Read the model definition and answer for the solid it produces. Units are mm, in the model's axes. A direction names the side the tool comes from. Round coordinates to 2 decimals unless told otherwise and drop trailing zeros. Order: outer loops, then holes, each group sorted by start corner. A loop starts at its lowest first (then second) coordinate and runs counter-clockwise, first axis right, second up. Notation, with made-up numbers: (-24, 49.5) - (20, 49.5) arc R28 ccw to (20, 69.5) - close; hole circle Ø7 at (67, 17.25). An arc over 180 degrees is marked (long way). Put each result on its own line as item: value. Start each with the question number.
Q1. Which of the six approach directions +Z, -Z, +X, -X, +Y, -Y give full straight-line access (tool end or side, diameter ignored) to faces 1 (the face through (0, 0, 0)), 2 (the face through (18, -10, 17)), 3 (the face through (-14.45, 9, 47.32)), 4 (the face through (-18, 0, 33)), 5 (the face through (-0.1, 10.6, 60))?
Q2. For a pull along X with two mould halves and no side action, classify faces 6 (the face through (14.45, -9, 47.32)), 7 (the face through (-23.651, -11.715, 47.025)), 8 (the face through (5, 0, 18)), 9 (the face through (18, 0, 33)) as pulls with the +X half, pulls with the -X half, needs draft (parallel to the pull), parting line crosses it, or undercut.
Q3. Each of these flat-tipped pins is pushed along its axis until it touches: pin 1 Ø10 at (x, z) = (21.5, 52.5) entering from -Y; pin 2 Ø5 at (x, y) = (21, -6.5) entering from +Z; pin 3 Ø8 at (y, z) = (-4, 43.5) entering from -X; pin 4 Ø10.5 at (y, z) = (2.5, 53) entering from +X (3 decimals). Where does it stop, or does it pass through?
Q4. Section D-D on z = 31 is taken. Give the vertices of the cut face in (x, y), then the cut area to 3 significant figures.
Q5. Section C-C on y = -2 is taken. Give the vertices of the cut face in (x, z).
Q6. Find the intervals of material crossed by line 1 along Y through (x, z) = (-24.5, 28); line 2 along Z through (x, y) = (-14, -5.25); line 3 along X through (y, z) = (-7, 4.5), in increasing order. Write a range as from..to.
Q7. Section B-B on z = 25 is taken. Give the vertices of the cut face in (x, y).
Q8. Section A-A on x = -11 is taken. Give the vertices of the cut face in (y, z), then the cut area to 3 significant figures.
from build123d import *

# Parameters (mm, degrees)
F0_W     = 60
F0_H     = 24
F1_DEPTH = 60
F2_W     = 31
F2_H     = 20
F5_DEPTH = 25
F4_W     = 20
F4_H     = 31
F6_DEPTH = 25
F3_W     = 20
F3_H     = 31
F7_DEPTH = 25
F8_SIZE2 = 25
F8_SIZE  = 12.5
F9_R     = 3.5
F10_R    = 1


with BuildPart() as f1:
    # F0 (on Top) → F1 (new body)
    with BuildSketch(Plane.XY):
        Rectangle(F0_W, F0_H)
    extrude(amount=F1_DEPTH)

    # F2 (on face) → F5 (cut)
    with BuildSketch(Plane.XY.offset(60)):
        Rectangle(F2_W, F2_H)
    extrude(amount=-F5_DEPTH, mode=Mode.SUBTRACT)

    # F4 (on face) → F6 (cut)
    with BuildSketch(Plane(origin=(-30, 0, 0), x_dir=(0, -1, 0), z_dir=(-1, 0, 0))):
        with Locations((0, 17.5)):
            Rectangle(F4_W, F4_H)
    extrude(amount=-F6_DEPTH, mode=Mode.SUBTRACT)

    # F3 (on face) → F7 (cut)
    with BuildSketch(Plane.YZ.offset(30)):
        with Locations((0, 17.5)):
            Rectangle(F3_W, F3_H)
    extrude(amount=-F7_DEPTH, mode=Mode.SUBTRACT)

    # F8
    f8_edges = [f1.edges().sort_by_distance(p)[0] for p in [
        (30, 0, 60),
        (-30, 0, 60),
    ]]
    f8_side = f1.faces().sort_by_distance((0, -11.35378, 60))[0]
    chamfer(f8_edges, length=F8_SIZE, length2=F8_SIZE2, reference=f8_side)

    # F9
    f9_edges = [f1.edges().sort_by_distance(p)[0] for p in [
        (-17.5, 10, 33),
        (-17.5, -10, 33),
        (-17.5, -10, 2),
        (-17.5, 10, 2),
        (15.5, -10, 47.5),
        (15.5, 10, 47.5),
        (-15.5, 10, 47.5),
        (-15.5, -10, 47.5),
        (17.5, -10, 2),
        (17.5, -10, 33),
        (17.5, 10, 33),
        (17.5, 10, 2),
    ]]
    fillet(f9_edges, radius=F9_R)

    # F10
    f10_edges = [f1.edges().sort_by_distance(p)[0] for p in [
        (-30, -12, 17.5),
        (-23.75, -12, 47.5),
        (0, -12, 0),
        (0, -12, 60),
        (30, -12, 17.5),
        (23.75, -12, 47.5),
        (30, 12, 17.5),
        (23.75, 12, 47.5),
        (0, 12, 0),
        (0, 12, 60),
        (-30, 12, 17.5),
        (-23.75, 12, 47.5),
        (30, 0, 0),
        (-30, 0, 0),
        (-17.5, 0, 60),
        (-30, 0, 35),
        (17.5, 0, 60),
        (30, 0, 35),
    ]]
    fillet(f10_edges, radius=F10_R)


solid = f1.part
Findings:
1. face 1: -Z, +X, -X, +Y, -Y
1. face 2: +X
1. face 3: +Z
1. face 4: -X
1. face 5: +Z, +X, -X, +Y, -Y
2. face 6: undercut
2. face 7: pulls with the -X half
2. face 8: pulls with the +X half
2. face 9: needs draft
3. pin 1: y = -12
3. pin 2: z = 58
3. pin 3: x = -27.75
3. pin 4: x = 23.625
4. outline: (-30, -11) arc R1 ccw to (-29, -12) - (29, -12) arc R1 ccw to (30, -11) - (30, -9.66) - (5, -9.66) - (5, 9.66) - (30, 9.66) - (30, 11) arc R1 ccw to (29, 12) - (-29, 12) arc R1 ccw to (-30, 11) - (-30, 9.66) - (-5, 9.66) - (-5, -9.66) - (-30, -9.66) - close
4. area: 473 mm2
5. outline: (-30, 1) arc R1 ccw to (-29, 0) - (29, 0) arc R1 ccw to (30, 1) - (30, 2) - (5, 2) - (5, 33) - (30, 33) - (30, 34.76) arc R1 ccw to (29.89, 35.21) - (17.78, 59.45) arc R1 ccw to (16.88, 60) - (15.5, 60) - (15.5, 35) - (-15.5, 35) - (-15.5, 60) - (-16.88, 60) arc R1 ccw to (-17.78, 59.45) - (-29.89, 35.21) arc R1 ccw to (-30, 34.76) - (-30, 33) - (-5, 33) - (-5, 2) - (-30, 2) - close
6. line 1: -12..-10, 10..12
6. line 2: 0..2, 33..35
6. line 3: -5..5
7. outline: (-30, -11) arc R1 ccw to (-29, -12) - (29, -12) arc R1 ccw to (30, -11) - (30, -10) - (5, -10) - (5, 10) - (30, 10) - (30, 11) arc R1 ccw to (29, 12) - (-29, 12) arc R1 ccw to (-30, 11) - (-30, 10) - (-5, 10) - (-5, -10) - (-30, -10) - close
8. outline: (-12, 1) arc R1 ccw to (-11, 0) - (11, 0) arc R1 ccw to (12, 1) - (12, 59) arc R1 ccw to (11, 60) - (10, 60) - (10, 35) - (-10, 35) - (-10, 60) - (-11, 60) arc R1 ccw to (-12, 59) - close; hole (-10, 5.5) arc R3.5 ccw to (-6.5, 2) - (6.5, 2) arc R3.5 ccw to (10, 5.5) - (10, 29.5) arc R3.5 ccw to (6.5, 33) - (-6.5, 33) arc R3.5 ccw to (-10, 29.5) - close
8. area: 330 mm2
